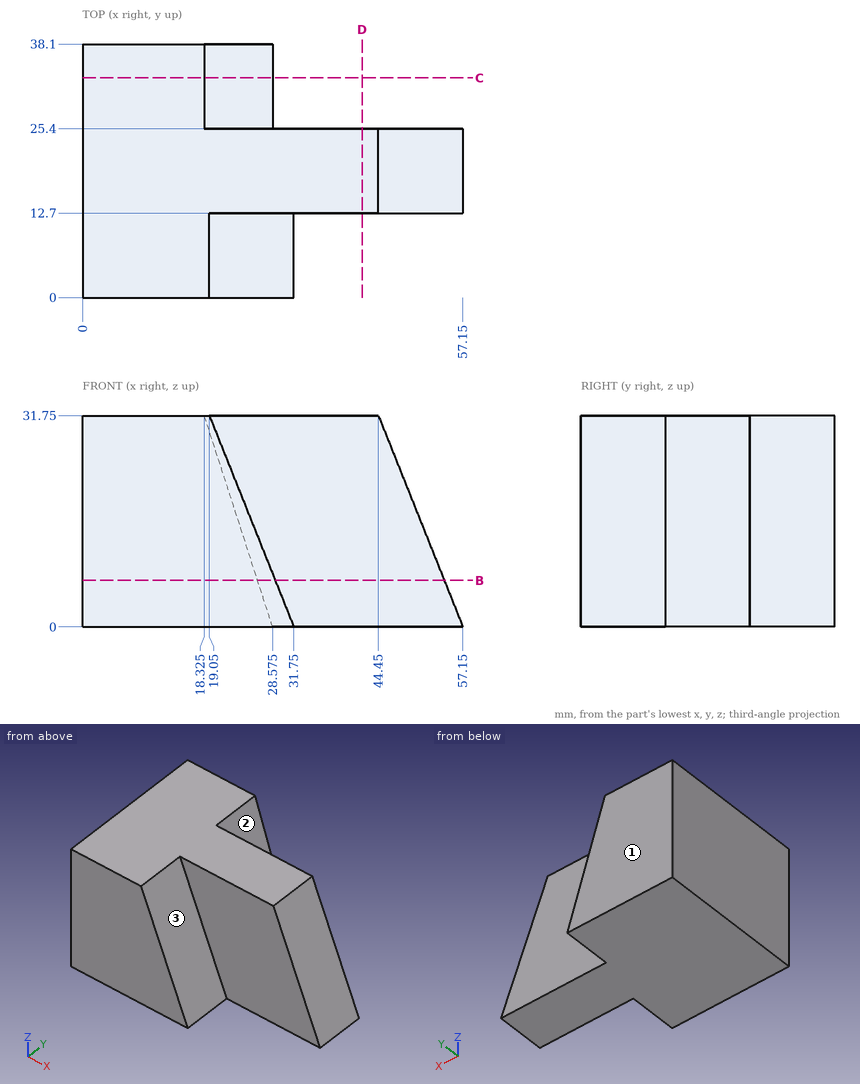
Job drawing, mm, ordinate dimensions from the low corner. One solid piece. A direction names the side the tool comes from. Coordinates: 2 decimals unless noted, no trailing zeros. Write each loop counter-clockwise with the first axis right and the second up, starting at its lowest first coordinate (ties: lowest second). Pieces come first, ordered by that corner, then holes. Notation, with made-up numbers: (9.5, 85) -> (39.5, 85) arc R22 cw to (39.5, 101) -> close; hole circle Ø11 at (-4, 42). An arc over 180 degrees is marked (long way). Use CSV: the item, a comma, the result in double quotes. Start each with the question number.
Item 1: Band-saw the part on B-B, the plane z = 7. Write the cut outline in (x, y) (3 decimals).
Item 2: Tool access for the marked faces 1, 2 and 3: list every direction of +Z, -Z, +X, -X, +Y, -Y with a clear straight run to the whole face (end or side of a thin tool).
Item 3: Drop flat-ended pins along their axis: P1, Ø5, axis at y = 19, z = 22.5, coming from the -X side; P2, Ø1, axis at x = 44, y = 11.5, coming from the +Z side; P3, Ø1.5, axis at x = 40, z = 22.5, coming from the -Y side; P4, Ø9.5, axis at x = 28.5, z = 22, coming from the +Y side. Give the stop position or say it passes through.
Item 4: Band-saw the part on C-C, the plane y = 33. Write the cut outline in (x, z) (3 decimals).
Item 5: Band-saw the part on D-D, the plane x = 42. Write the cut outline in (y, z).
Item 6: Wall check: probe 1 along Y at (x, z) = (48, 3); probe 2 along X at (y, z) = (23, 18); probe 3 along X at (y, z) = (32, 20). Give the ranges that are in metal, low to high.
Response values:
1,outline,"(0, 0) -> (28.95, 0) -> (28.95, 12.7) -> (54.35, 12.7) -> (54.35, 25.4) -> (26.315, 25.4) -> (26.315, 38.1) -> (0, 38.1) -> close"
2,face 1,"+Z, -Z, +X, -X, +Y"
2,face 2,"+Z, +X, +Y"
2,face 3,"+Z, +X, -Y"
3,P1,"stops at x = 0"
3,P2,"passes through"
3,P3,"stops at y = 12.7"
3,P4,"stops at y = 25.4"
4,outline,"(0, 0) -> (28.575, 0) -> (18.325, 31.75) -> (0, 31.75) -> close"
5,outline,"(12.7, 0) -> (25.4, 0) -> (25.4, 31.75) -> (12.7, 31.75) -> close"
6,probe 1,"y = 12.7 to 25.4"
6,probe 2,"x = 0 to 49.95"
6,probe 3,"x = 0 to 22.12"
